from build123d import *

# Parameters (mm, degrees)
F0_W        = 79.0347680449
F0_H        = 51.5021067113
F1_DEPTH    = 21.9734124839
F2_T1_DEPTH = 76.5021067113
F3_T        = 2.5


# Not quite as in the source:
# - a fillet or chamfer that OpenCascade refuses, or shapes differently, is made with other operations: its cross-section is extruded or revolved along the edge and cut away or added
# - a shell that OpenCascade refuses in one call is made with other operations: the cavity is built on its own and cut out


with BuildPart() as f1:
    # F0 (on Top) → F1 (new body)
    with BuildSketch(Plane.XY):
        with Locations((-4.2740143836, 13.997332193)):
            Rectangle(F0_W, F0_H)
    extrude(amount=F1_DEPTH)

    # F2: fillet of radius 5 on 2 edges, made by hand

    # F2_s2 → F2_t1 (cut)
    with BuildSketch(Plane.XZ.offset(-52.2483855486)):
        with BuildLine():
            add(Edge.make_bspline(
                [(-43.791398406, 16.9734124839), (-43.791398406, 21.9734124839), (-38.791398406, 21.9734124839)],
                knots=[0, 0, 0, 1, 1, 1], degree=2, weights=[1, 1, 1]))
            Line((-38.791398406, 21.9734124839), (-43.791398406, 21.9734124839))
            Line((-43.791398406, 21.9734124839), (-43.791398406, 16.9734124839))
        make_face()
        with BuildLine():
            add(Edge.make_bspline(
                [(35.2433696389, 16.9734124839), (35.2433696389, 21.9734124839), (30.2433696389, 21.9734124839)],
                knots=[0, 0, 0, 1, 1, 1], degree=2, weights=[1, 1, 1]))
            Line((30.2433696389, 21.9734124839), (35.2433696389, 21.9734124839))
            Line((35.2433696389, 21.9734124839), (35.2433696389, 16.9734124839))
        make_face()
    extrude(amount=F2_T1_DEPTH, mode=Mode.SUBTRACT)

    # F3: shell of thickness 2.5, made by hand


with BuildPart() as f3_core1:
    # F3_t2: copy of F1
    add(f1.part)

    # the walls: a layer under each face that stays
    f3_faces = [f3_core1.faces().sort_by_distance(p)[0] for p in [
        (-43.791398406, 13.997332193, 8.4867062419),
        (-4.2740143836, 13.997332193, 0),
        (-42.541398406, 13.997332193, 20.7234124839),
        (-4.2740143836, 39.7483855486, 10.986706242),
        (35.2433696389, 13.997332193, 8.4867062419),
        (33.9933696389, 13.997332193, 20.7234124839),
    ]]
    thicken(f3_faces, amount=-F3_T, mode=Mode.SUBTRACT)


with BuildPart() as f1_1:
    add(f1.part)

    # what is left inside the walls is the cavity
    f3_cavity = [f3_core1.part.solids().sort_by_distance(p)[0] for p in [
        (-4.274014, 4.580314, 2.525),
    ]]
    add(f3_cavity, mode=Mode.SUBTRACT)


solid = f1_1.part
For this review, take the finished solid that the model builds, in its own axes (mm). A direction names the side the tool comes from. Round coordinates to 2 decimals unless told otherwise and drop trailing zeros. Loops run counter-clockwise (first coordinate to the right, second up) from the corner with the lowest first, then second, coordinate; pieces in that order, holes last. Notation, with made-up numbers: (-2, 65) - (54, 65) arc R28 cw to (54, 98) - close; hole circle Ø9 at (-25.5, 67). An arc over 180 degrees is marked (long way). Put each result on its own line as item: value. Start each with the question number.
1. Mouldability with a two-part tool opening along X and no side actions: class faces 1 (the flat face through (-5, 39.748, 11)), 2 (the flat face through (30.243, 12, 21)), 3 (the flat face through (-5, 37.248, 12)), 4 (the flat face through (35.243, 14, 8)) as +X half, -X half, draft (parallel to the pull), parting line (faces both ways), or undercut.
2. Insertion check: P1, Ø5, axis at x = 5, z = 14, coming from the -Y side; P2, Ø3, axis at y = 13, z = 20.5, coming from the -X side; P3, Ø12, axis at x = -2, y = -2, coming from the +Z side. Each pin has a flat end and moves straight along its axis. Give the tip position at first contact, or say it passes through.
3. Consider section B-B on x = -11. State the section outline as (y, z) points, plus the area to 3 significant figures.
4. For faces 5 (the flat face through (-38.791, 12, 21)), 6 (the flat face through (32.743, 12, 10)), 7 (the flat face through (-5, 14, 0)), list the 3-axis set-ups (+Z, -Z, +X, -X, +Y, -Y) from which the entire face can be reached by the end or side of a thin tool; tool diameter is ignored.
5. Consider section A-A on z = 14.75. State the section outline as (x, y) points, plus the area to 3 significant figures.
6. For probe 1 along X at (y, z) = (15, 15); probe 2 along Z at (x, y) = (13.5, 30); probe 3 along Y at (x, z) = (-22, 20.25), list the stretches that pass through material, from the lowest coordinate up. Write a range as [from, to].
Result sheet:
1. face 1: draft
1. face 2: undercut
1. face 3: undercut
1. face 4: +X half
2. P1: y = 37.25
2. P2: x = -43.53
2. P3: z = 2.5
3. outline: (-11.75, 0) - (39.75, 0) - (39.75, 21.97) - (37.25, 21.97) - (37.25, 2.5) - (-11.75, 2.5) - close
3. area: 177 mm^2
4. face 5: +Z, -Y
4. face 6: -Y
4. face 7: -Z, +X, -X, +Y, -Y
5. outline: (-43.79, -11.75) - (-41.29, -11.75) - (-41.29, 37.25) - (32.74, 37.25) - (32.74, -11.75) - (35.24, -11.75) - (35.24, 39.75) - (-43.79, 39.75) - close
5. area: 443 mm^2
6. probe 1: [-43.79, -41.29], [32.74, 35.24]
6. probe 2: [0, 2.5]
6. probe 3: [37.25, 39.75]
